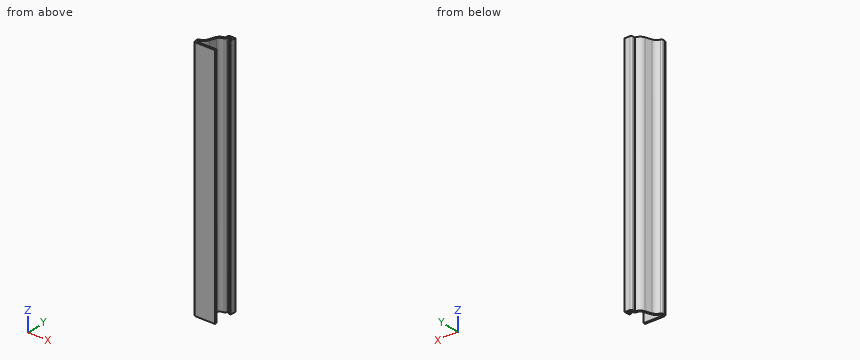
```python
from build123d import *

# Parameters (mm, degrees)
EXTRUDE_THIN1_DEPTH = 142.875
FILLET1_R           = 1.016


with BuildPart() as part:
    # Sketch1 → Extrude-Thin1 (new body)
    with BuildSketch(Plane.XY):
        with BuildLine():
            Line((-0.396875, 0), (-12.7, 0))
            Line((-12.7, 0), (-12.7, 3.175))
            ThreePointArc((-12.7, 3.175), (-10.421749313, 3.894049957), (-8.969036168, 5.790647844))
            Line((-8.969036168, 5.790647844), (-7.699713832, 9.290602156))
            ThreePointArc((-7.699713832, 9.290602156), (-6.247000687, 11.187200043), (-3.96875, 11.90625))
            Line((-3.96875, 11.90625), (-3.96875, 14.2875))
            Line((-3.96875, 14.2875), (0, 14.2875))
            Line((0, 14.2875), (-0.396875, 11.137402345))
            Line((-0.396875, 11.137402345), (-1.40490625, 11.264402345))
            Line((-1.40490625, 11.264402345), (-1.152035714, 13.2715))
            Line((-1.152035714, 13.2715), (-2.95275, 13.2715))
            Line((-2.95275, 13.2715), (-2.95275, 10.70994956))
            ThreePointArc((-2.95275, 10.70994956), (-5.215232033, 10.614254584), (-6.744587091, 8.944208004))
            Line((-6.744587091, 8.944208004), (-8.013909427, 5.444253692))
            ThreePointArc((-8.013909427, 5.444253692), (-9.435411883, 3.376762213), (-11.684, 2.263639698))
            Line((-11.684, 2.263639698), (-11.684, 1.016))
            Line((-11.684, 1.016), (-0.396875, 1.016))
            Line((-0.396875, 1.016), (-0.396875, 0))
        make_face()
    extrude(amount=-EXTRUDE_THIN1_DEPTH)

    # Fillet1
    fillet1_edges = [part.edges().sort_by_distance(p)[0] for p in [
        (-2.95275, 10.70994956, -71.4375),
        (-12.7, 0, -71.4375),
        (-12.7, 3.175, -71.4375),
        (-3.96875, 14.2875, -71.4375),
    ]]
    fillet(fillet1_edges, radius=FILLET1_R)


solid = part.part
```
Work out the finished part from the listing and answer in its coordinate system (mm). Give positions to 0.01 mm unless a question says otherwise; leave off trailing zeros. Loops run counter-clockwise (first coordinate to the right, second up) from the corner with the lowest first, then second, coordinate; pieces in that order, holes last. Notation, with made-up numbers: (-22, 41) - (-9, 41) arc R29 cw to (-9, 73) - close; hole circle Ø4 at (74.25, 71.25). An arc over 180 degrees is marked (long way). One line per question, with ' | ' between items.
(1) The part is cut by section B-B (x = -10.25). Write down the section's boundary in (y, z) (1 decimal).
Recorded:
outline: (0, -142.9) - (1, -142.9) - (1, 0) - (0, 0) - close; (2.8, -142.9) - (4, -142.9) - (4, 0) - (2.8, 0) - close
(2) The part is cut by section A-A (z = -107.5). Write down the section's boundary in (x, y), then the cut area to 3 significant figures.
Recorded:
outline: (-12.7, 1.02) arc R1.02 ccw to (-11.68, 0) - (-0.4, 0) - (-0.4, 1.02) - (-11.68, 1.02) - (-11.68, 2.26) arc R4.98 ccw to (-8.01, 5.44) - (-6.74, 8.94) arc R2.95 cw to (-3.97, 10.89) arc R1.02 ccw to (-2.95, 11.91) - (-2.95, 13.27) - (-1.15, 13.27) - (-1.4, 11.26) - (-0.4, 11.14) - (0, 14.29) - (-2.95, 14.29) arc R1.02 ccw to (-3.97, 13.27) - (-3.97, 11.91) arc R3.97 ccw to (-7.7, 9.29) - (-8.97, 5.79) arc R3.97 cw to (-11.89, 3.26) arc R1.02 ccw to (-12.7, 2.26) - close | area: 35.0 mm²
(3) Each of these flat-tipped pins is pushed along its axis until it touches: pin 1 Ø3.5 at (x, z) = (-6.5, -56.5) entering from +Y; pin 2 Ø0.7 at (y, z) = (13, -102.5) entering from -X; pin 3 Ø0.5 at (y, z) = (0.5, -94.5) entering from +X. Where does it stop, or does it pass through?
Recorded:
pin 1: stops at y = 11.83 | pin 2: stops at x = -3.97 | pin 3: stops at x = -0.4
(4) The part is cut by section C-C (y = 7). Write down the section's boundary in (x, z) (3 decimals).
Recorded:
outline: (-8.53, -142.875) - (-7.45, -142.875) - (-7.45, 0) - (-8.53, 0) - close
(5) Straight lines are drawn through the part: probe 1 along Y at (x, z) = (-2.25, -66); probe 2 along Y at (x, z) = (-0.5, -52.5); probe 3 along X at (y, z) = (1.25, -21). For each, find the intervals that lie inside material, in ascending order.
Recorded:
probe 1: y = 0 to 1.02, 13.27 to 14.29 | probe 2: y = 0 to 1.02, 11.15 to 14.29 | probe 3: x = -12.7 to -11.68
